The figure shows three views and two pictorial views of one solid part (mm, origin at its lowest corner). Answer the questions. Coordinates: 2 decimals unless noted, no trailing zeros. Write each loop counter-clockwise with the first axis right and the second up, starting at its lowest first coordinate (ties: lowest second). Pieces come first, ordered by that corner, then holes. Notation, with made-up numbers: M 22.25,-34.5 L 28.25,-34.5 A14 cw 28.25,-29.5 Z; hole C -10.75,48.5 d8. An arc over 180 degrees is marked long. Write item = value, one per line. Start each with the question number.
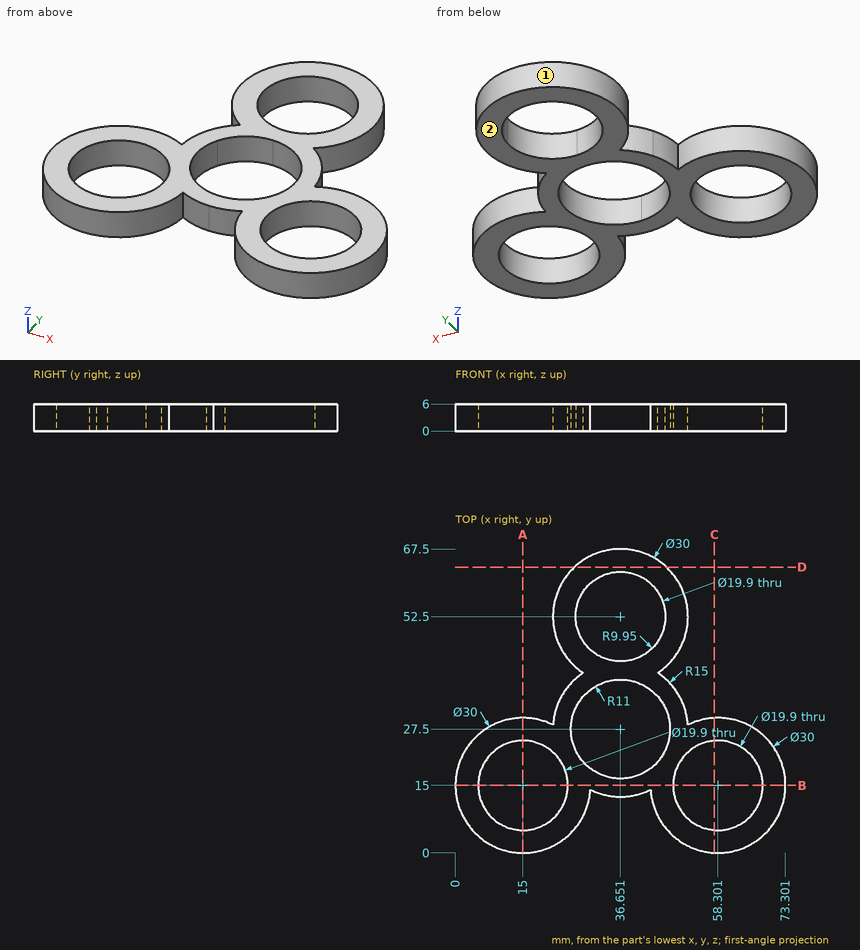
1. The part is cut by section C-C, the plane x = 57.5. Write down the section's boundary in (y, z).
2. The part is cut by section A-A, the plane x = 15. Write down the section's boundary in (y, z), and give its area (3 significant figures).
3. The part is cut by section B-B, the plane y = 15. Write down the section's boundary in (x, z).
4. Each of these flat-tipped pins is pushed along its axis until it touches: pin 1 (3 mm diameter, centred on y = 47, z = 1, fed in from +X); pin 2 (12 mm diameter, centred on x = 15, y = 15, fed in from +Z); pin 3 (2 mm diameter, centred on x = 48, z = 4, fed in from -Y). Where does it stop, or does it pass through?
5. Straight lines are drawn through the part: L1, parallel to X at y = 15.5, z = 4.4; L2, parallel to X at y = 15, z = 1.3; L3, parallel to Y at x = 15.5, z = 4.9. For each, find the intervals that lie inside material, in ascending order. Write a range as [from, to].
6. For a pull along Y with two mould halves and no side action, classify the marked faces 1 and 2 as pulls with the +Y half, pulls with the -Y half, needs draft (parallel to the pull), parting line crosses it, or undercut.
7. The part is cut by section D-D, the plane y = 63.5. Write down the section's boundary in (x, z).
Solution:
q1.outline = M 0.02,0 L 5.08,0 L 5.08,6 L 0.02,6 Z; M 24.92,0 L 29.98,0 L 29.98,6 L 24.92,6 Z
q2.outline = M 0,0 L 5.05,0 L 5.05,6 L 0,6 Z; M 24.95,0 L 30,0 L 30,6 L 24.95,6 Z
q2.area = 60.6 mm^2
q3.outline = M 0,0 L 5.05,0 L 5.05,6 L 0,6 Z; M 24.95,0 L 48.35,0 L 48.35,6 L 24.95,6 Z; M 68.25,0 L 73.3,0 L 73.3,6 L 68.25,6 Z
q4.pin_1 = 51.11
q4.pin_2 = through
q4.pin_3 = 3.23
q5.L1 = [0.01, 5.06], [24.94, 48.36], [68.24, 73.29]
q5.L2 = [0, 5.05], [24.95, 48.35], [68.25, 73.3]
q5.L3 = [0.01, 5.06], [24.94, 29.99]
q6.face_1 = undercut
q6.face_2 = needs draft
q7.outline = M 26.45,0 L 46.85,0 L 46.85,6 L 26.45,6 Z
